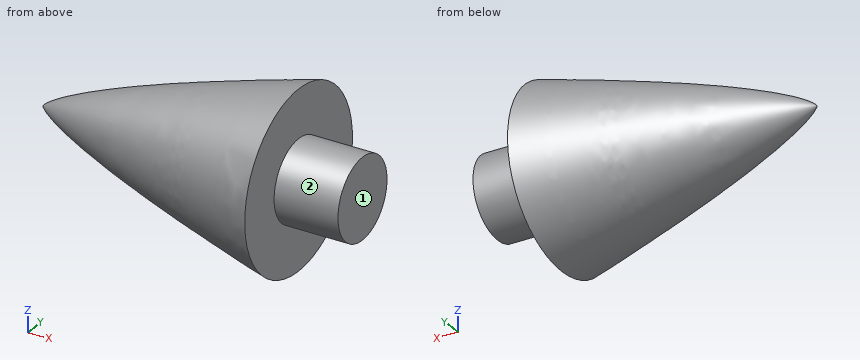
```python
from build123d import *

# Parameters (mm, degrees)
SKETCH5_W           = 40
SKETCH5_H           = 13.888133248
SKETCH6_R           = 6.32
BOSS_EXTRUDE1_DEPTH = 10


with BuildPart() as part:
    # Sketch4 → Revolve3 (revolve)
    with BuildSketch(Plane(origin=(0, 0, 0), x_dir=(1, 0, 0), z_dir=(0, 1, 0))):
        with BuildLine():
            Line((0, 0), (700, 0))
            Line((700, 0), (700, 92))
            add(Edge.make_bspline(
                [(0, 0), (0.00191147, 0.007452455), (0.006682771, 0.021975667), (0.020319911, 0.049405272), (0.053712312, 0.100813891), (0.106292543, 0.166564672), (0.179361524, 0.244890293), (0.321314168, 0.380305786), (0.489821471, 0.519272356), (0.682008296, 0.663619163), (0.97824001, 0.869271861), (1.381516871, 1.128290995), (2.087665161, 1.540864263), (3.352844681, 2.20038034), (5.559362022, 3.217605874), (9.551431072, 4.830778204), (16.8107271, 7.377330859), (28.917425512, 11.039410523), (45.357311817, 15.359469167), (65.219754515, 20.019307373), (92.239595195, 25.797411612), (124.65879636, 32.080212127), (162.600367905, 38.763077948), (206.074460711, 45.728609064), (249.632824355, 52.143059314), (293.258988419, 58.07761177), (336.942021596, 63.576842057), (380.674593437, 68.666747534), (424.45146039, 73.360146302), (468.268944021, 77.658075094), (512.124428867, 81.549646326), (556.016196354, 85.009603585), (594.452384, 87.618355269), (627.419605801, 89.502855515), (653.668023827, 90.726417336), (671.057263835, 91.380719564), (685.081182637, 91.780411211), (693.605741334, 91.941702123), (697.868499327, 91.993335353), (700, 92)],
                knots=[0, 0, 0, 0, 0, 4.3185e-05, 8.637e-05, 0.000172741, 0.000345481, 0.000518222, 0.000690962, 0.001280476, 0.001578086, 0.001875696, 0.002727788, 0.00398729, 0.006196413, 0.009932334, 0.016447975, 0.028301339, 0.049639657, 0.081363194, 0.112451539, 0.143539883, 0.205716599, 0.267893307, 0.330070016, 0.392246725, 0.454423434, 0.516600142, 0.578776854, 0.640953563, 0.703130272, 0.765306983, 0.827483692, 0.889660402, 0.920748757, 0.951837113, 0.975918556, 0.987959278, 1, 1, 1, 1, 1], degree=4))
        make_face()
    revolve(axis=Axis((0, 0, 0), (1, 0, 0)))


with BuildPart() as body_2:
    # Sketch5 → Revolve5 (revolve)
    with BuildSketch(Plane.XY, mode=Mode.PRIVATE) as revolve5_sk:
        with Locations((20, 6.944066624)):
            Rectangle(SKETCH5_W, SKETCH5_H)
    revolve(revolve5_sk.sketch.rotate(Axis((0, 0, 0), (1, 0, 0)), 90), axis=Axis((0, 0, 0), (1, 0, 0)))

    # Combine1: intersect part
    add(part.part, mode=Mode.INTERSECT)

    # Sketch6 → Boss-Extrude1 (add)
    with BuildSketch(Plane(origin=(40, 0, 0), x_dir=(0, 0, -1), z_dir=(1, 0, 0))):
        with Locations(Location((0, 0, 0), (0, 0, 180))):
            Circle(SKETCH6_R)
    extrude(amount=BOSS_EXTRUDE1_DEPTH)


solid = body_2.part
```
Geometry check sheet. Reference: the model listing, model coordinates, mm. Face numbers are marked on the shaded views. A direction names the side the tool comes from. Round coordinates to 2 decimals unless told otherwise and drop trailing zeros. Loops run counter-clockwise (first coordinate to the right, second up) from the corner with the lowest first, then second, coordinate; pieces in that order, holes last. Notation, with made-up numbers: (68.25, -25) - (88.25, -25) arc R16 ccw to (88.25, 6) - close; hole circle Ø9 at (-38, -17.75). An arc over 180 degrees is marked (long way). Write item = value, one per line. Start each with the question number.
1. Set-up check for the marked faces 1 and 2: record each of +Z, -Z, +X, -X, +Y, -Y from which the full face is reachable in a straight line by a thin tool's end or side.
2. Thickness scan on line 1 (Y direction, x = 36.5, z = 8.5); line 2 (Z direction, x = 40.5, y = -3.75); line 3 (Z direction, x = 47, y = -3). Record the ranges inside material, lowest first.
3. Section check A-A on x = 43. Enter the section's corners in (y, z).
4. Depth check by flat-ended pin: pin 1 (1.5 mm diameter, centred on x = 40, z = 6.5, fed in from +Y); pin 2 (1 mm diameter, centred on x = 25, y = -2.5, fed in from -Z); pin 3 (2 mm diameter, centred on x = 25.5, y = 7, fed in from -Z). Enter the tip coordinate at first touch or a pass-through.
Working result:
q1.face_1 = +Z, -Z, +X, +Y, -Y
q1.face_2 = +X
q2.line_1 = -9.8 to 9.8
q2.line_2 = -5.09 to 5.09
q2.line_3 = -5.56 to 5.56
q3.outline = circle Ø12.64 at (0, 0)
q4.pin_1 = 12.64
q4.pin_2 = -9.66
q4.pin_3 = -8.01
